```python
from build123d import *

# Parameters (mm, degrees)
BOSS_EXTRUDE1_DEPTH = 15
SKETCH2_R           = 3
CUT_EXTRUDE1_DEPTH  = 15
SKETCH3_R           = 1.5
CUT_EXTRUDE2_DEPTH  = 15


with BuildPart() as part:
    # Sketch1 → Boss-Extrude1 (new body)
    with BuildSketch(Plane.XY):
        with BuildLine():
            Line((9, 0), (3, 0))
            ThreePointArc((3, 0), (0, -3), (-3, 0))
            Line((-3, 0), (-9, 0))
            ThreePointArc((-9, 0), (0, -9), (9, 0))
        make_face()
    extrude(amount=BOSS_EXTRUDE1_DEPTH)

    # Sketch2 → Cut-Extrude1 (cut)
    with BuildSketch(Plane(origin=(0, -2, 0), x_dir=(1, 0, 0), z_dir=(0, 1, 0))):
        with Locations(Location((5.5, -7.5, 0), (0, 0, 270))):
            Circle(SKETCH2_R)
    cut_extrude1 = extrude(amount=-CUT_EXTRUDE1_DEPTH, mode=Mode.SUBTRACT)

    # Sketch3 → Cut-Extrude2 (cut)
    with BuildSketch(Plane.XZ.offset(2)):
        with Locations(Location((5.5, 7.5, 0), (0, 0, 270))):
            Circle(SKETCH3_R)
    cut_extrude2 = extrude(amount=-CUT_EXTRUDE2_DEPTH, mode=Mode.SUBTRACT)

    # Mirror1: Cut-Extrude1, Cut-Extrude2 across plane
    add(cut_extrude1.mirror(Plane(origin=(0, 0, 0), x_dir=(0, 0, 1), z_dir=(1, 0, 0))), mode=Mode.SUBTRACT)
    add(cut_extrude2.mirror(Plane(origin=(0, 0, 0), x_dir=(0, 0, 1), z_dir=(1, 0, 0))), mode=Mode.SUBTRACT)


solid = part.part
```
Input: part model. Units: mm. Frame: model coordinates. A direction names the side the tool comes from. Round coordinates to 2 decimals unless told otherwise and drop trailing zeros. Order: outer loops, then holes, each group sorted by start corner. A loop starts at its lowest first (then second) coordinate and runs counter-clockwise, first axis right, second up. Notation, with made-up numbers: (19.5, -25) - (46.5, -25) arc R20 ccw to (46.5, 10) - close; hole circle Ø5 at (79.5, 49). An arc over 180 degrees is marked (long way). Answer in a Markdown table with one row per item.
Item 1: Pin query (flat end, axial travel): pin 1 (1.8 mm diameter, centred on x = -6, z = 6.5, fed in from -Y); pin 2 (1 mm diameter, centred on y = -1.5, z = 11, fed in from +X); pin 3 (4 mm diameter, centred on y = -7, z = 2.5, fed in from -X). Return the tip coordinate at first contact, or that it passes through.
Model answer:
| item | result |
|---|---|
| pin 1 | stops at y = -2 |
| pin 2 | stops at x = 8.94 |
| pin 3 | stops at x = -7.48 |
Item 2: Section query C-C (y = -1). Return the cut outline in (x, z), then the cut area to 3 significant figures.
Model answer:
| item | result |
|---|---|
| outline | (-8.94, 0) - (-2.83, 0) - (-2.83, 15) - (-8.94, 15) - close; (2.83, 0) - (8.94, 0) - (8.94, 15) - (2.83, 15) - close; hole circle Ø3 at (-5.5, 7.5); hole circle Ø3 at (5.5, 7.5) |
| area | 169 mm² |
Item 3: Line query: line 1 (Z direction, x = -5.5, y = -0.95); line 2 (Y direction, x = 7.25, z = 7.75); line 3 (X direction, y = -1.25, z = 7.5). Output: solid intervals per line, ascending.
Model answer:
| item | result |
|---|---|
| line 1 | z = 0 to 6, 9 to 15 |
| line 2 | y = -2 to 0 |
| line 3 | x = -8.91 to -7, -4 to -2.73, 2.73 to 4, 7 to 8.91 |
Item 4: Reachability of faces 1 (the flat face through (-4, -2, 9)), 2 (the flat face through (0, -4, 15)) from +Z, -Z, +X, -X, +Y, -Y: full face, straight path, thin tool, end or side. Return the list, or none.
Model answer:
| item | result |
|---|---|
| face 1 | -Y |
| face 2 | +Z, +X, -X, +Y, -Y |
Item 5: Mould query, pull axis X, two halves, no side actions, for faces 3 (the cylindrical face through (0, -9, 7)), 4 (the flat face through (7.4, 0, 7.4)), 5 (the flat face through (4, -2, 9)). Classes: released by +X, released by -X, zero draft, split by the parting line, or undercut.
Model answer:
| item | result |
|---|---|
| face 3 | split by the parting line |
| face 4 | zero draft |
| face 5 | undercut |
Item 6: Section query B-B (z = 7.75). Return the cut outline in (x, y).
Model answer:
| item | result |
|---|---|
| outline | (-9, 0) arc R9 ccw to (-8.49, -2.99) - (-8.49, -2) - (-6.98, -2) - (-6.98, 0) - close; (-4.02, -2) - (-2.51, -2) - (-2.51, -8.64) arc R9 ccw to (2.51, -8.64) - (2.51, -2) - (4.02, -2) - (4.02, 0) - (3, 0) arc R3 cw to (-3, 0) - (-4.02, 0) - close; (6.98, -2) - (8.49, -2) - (8.49, -2.99) arc R9 ccw to (9, 0) - (6.98, 0) - close |
Item 7: Section query A-A (x = -4.5). Return the cut outline in (y, z).
Model answer:
| item | result |
|---|---|
| outline | (-7.79, 0) - (0, 0) - (0, 6.38) - (-2, 6.38) - (-2, 4.67) - (-7.79, 4.67) - close; (-7.79, 10.33) - (-2, 10.33) - (-2, 8.62) - (0, 8.62) - (0, 15) - (-7.79, 15) - close |
Item 8: Section query D-D (y = -4.25). Return the cut outline in (x, z).
Model answer:
| item | result |
|---|---|
| outline | (-7.93, 0) - (7.93, 0) - (7.93, 5.75) arc R3 cw (long way) to (7.93, 9.25) - (7.93, 15) - (-7.93, 15) - (-7.93, 9.25) arc R3 cw (long way) to (-7.93, 5.75) - close |
